Verification items for the finished model (mm, model axes). Face numbers are marked on the shaded views. A direction names the side the tool comes from. Coordinates: 2 decimals unless noted, no trailing zeros. Order: outer loops, then holes, each group sorted by start corner. A loop starts at its lowest first (then second) coordinate and runs counter-clockwise, first axis right, second up. Notation, with made-up numbers: (45, 17.5) -> (72, 17.5) arc R19 ccw to (72, 42.5) -> close; hole circle Ø10 at (87.5, -16.75). An arc over 180 degrees is marked (long way). Use CSV: the item, a comma, the result in double quotes. Start each with the question number.
1) Sectioned sample at C-C on x = -0.5. Record the boundary of the cut face in (y, z).
2) Go/stop test with flat-tipped pins: pin 1 (8 mm diameter, centred on x = 3, y = -8.5, fed in from -Z); pin 2 (14 mm diameter, centred on x = 19.5, z = 12.5, fed in from +Y); pin 3 (10 mm diameter, centred on x = 19, z = 3.5, fed in from -Y). Record where each tip stops, or that it passes through.
3) Scan lines: line 1 along X through (y, z) = (-19, 5); line 2 along Y through (x, z) = (-4.5, 20.5); line 3 along Z through (x, y) = (20, -3). Record each from-to range of solid material in increasing order.
4) Sectioned sample at D-D on y = 15. Record the boundary of the cut face in (x, z), then the cut area to 3 significant figures.
5) Sectioned sample at A-A on y = -11.5. Record the boundary of the cut face in (x, z), then the cut area to 3 significant figures.
6) Sectioned sample at B-B on z = 19. Record the boundary of the cut face in (x, y).
7) Tool access check on the marked faces 1, 2 and 3. Record the directions out of +Z, -Z, +X, -X, +Y, -Y that give a thin tool (end or side, any length) a straight path to the whole face; none if there is none.
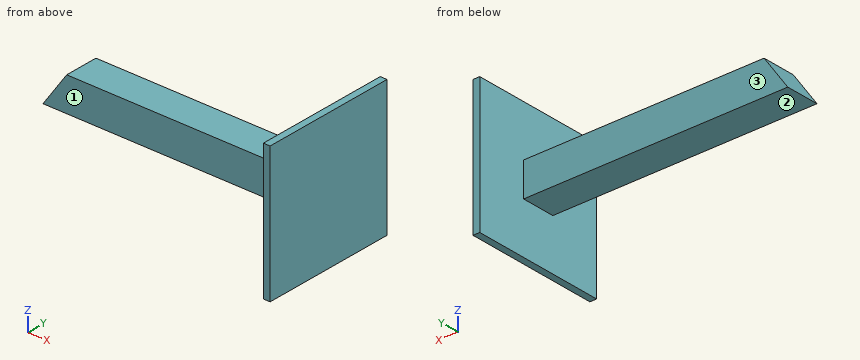
from build123d import *

# Parameters (mm, degrees)
F0_W     = 101.6
F0_H     = 12.7
F1_DEPTH = 12.7
F3_DEPTH = 25.4
F4_W     = 12.7
F4_H     = 12.7
F5_DEPTH = 2.54
F7_DEPTH = 2.54


with BuildPart() as f1:
    # F0 (on Front) → F1 (new body)
    with BuildSketch(Plane.XZ):
        with Locations((7.6688484669, 14.4629018217)):
            Rectangle(F0_W, F0_H)
    extrude(amount=F1_DEPTH)

    # F2 (on face) → F3 (cut)
    with BuildSketch(Plane.XZ.offset(12.7)):
        Polygon((-43.1311515331, 20.8129018217), (-43.1311515331, 8.1129018217), (-34.2385157979, 20.8129018217), align=None)
    extrude(amount=-F3_DEPTH, mode=Mode.SUBTRACT)

    # F4 (on face) → F5 (cut)
    with BuildSketch(Plane.YZ.offset(58.4688484669)):
        with Locations((-6.35, 14.4629018217)):
            Rectangle(F4_W, F4_H)
    extrude(amount=-F5_DEPTH, mode=Mode.SUBTRACT)

    # F6 (on face) → F7 (join)
    with BuildSketch(Plane.YZ.offset(55.9288484669)):
        Polygon((-31.75, 39.8629018217), (-31.75, 20.8129018217), (-31.75, -10.9370981783), (19.05, -10.9370981783), (19.05, 39.8629018217), align=None)
    extrude(amount=F7_DEPTH)


solid = f1.part
Answers follow:
1,outline,"(-12.7, 8.11) -> (0, 8.11) -> (0, 20.81) -> (-12.7, 20.81) -> close"
2,pin 1,"stops at z = 8.11"
2,pin 2,"stops at y = 0"
2,pin 3,"stops at y = -12.7"
3,line 1,"x = 55.93 to 58.47"
3,line 2,"y = -12.7 to 0"
3,line 3,"z = 8.11 to 20.81"
4,outline,"(55.93, -10.94) -> (58.47, -10.94) -> (58.47, 39.86) -> (55.93, 39.86) -> close"
4,area,"129 mm²"
5,outline,"(-43.13, 8.11) -> (55.93, 8.11) -> (55.93, -10.94) -> (58.47, -10.94) -> (58.47, 39.86) -> (55.93, 39.86) -> (55.93, 20.81) -> (-34.24, 20.81) -> close"
5,area,"1,330 mm²"
6,outline,"(-35.51, -12.7) -> (55.93, -12.7) -> (55.93, -31.75) -> (58.47, -31.75) -> (58.47, 19.05) -> (55.93, 19.05) -> (55.93, 0) -> (-35.51, 0) -> close"
7,face 1,"+Z, -Z, -X, -Y"
7,face 2,"-Z, -X, +Y, -Y"
7,face 3,"+Z, -Z, -X, +Y"
